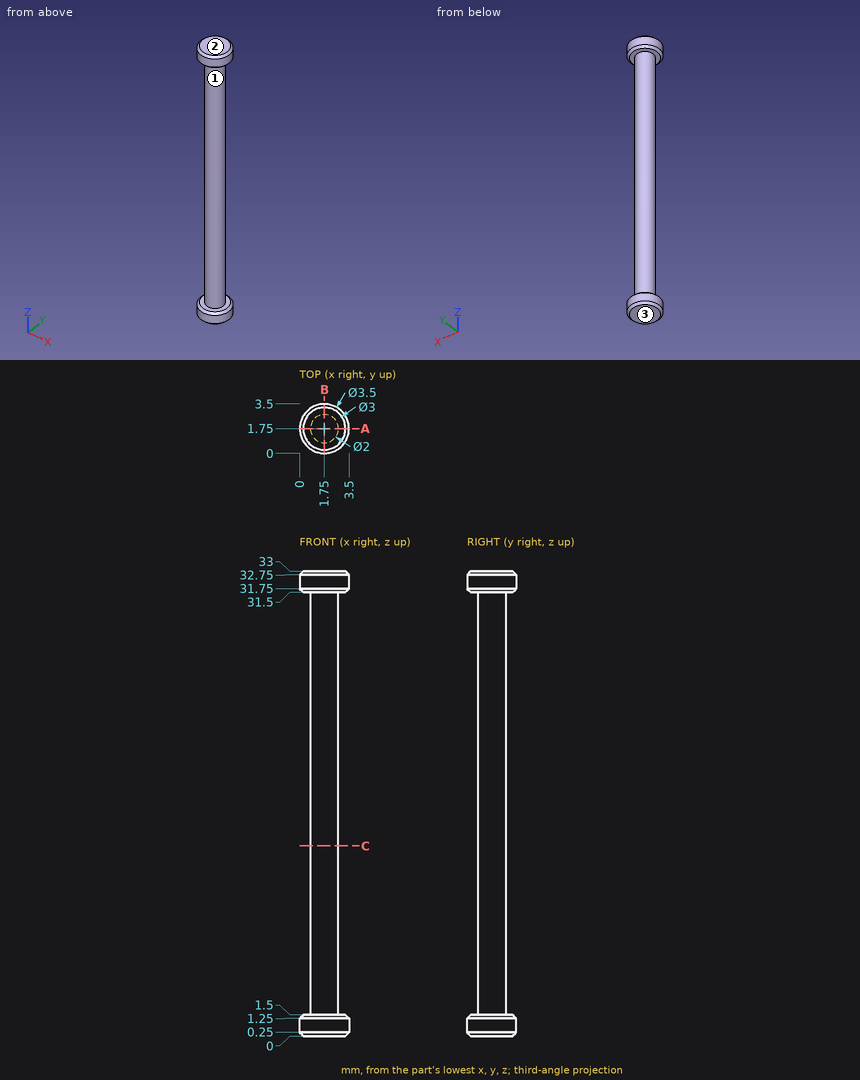
Here's the drawing with two shaded views (mm, measured from the low corner). I have some questions. Round coordinates to 2 decimals unless told otherwise and drop trailing zeros. Loops run counter-clockwise (first coordinate to the right, second up) from the corner with the lowest first, then second, coordinate; pieces in that order, holes last. Notation, with made-up numbers: (17.5, 82.25) - (64.5, 82.25) arc R15 ccw to (64.5, 109.25) - close; hole circle Ø8 at (-31, -21.75). An arc over 180 degrees is marked (long way). Write item = value, one per line.
1) Imagine slicing it at C-C (z = 13.5). Please give me the cut outline in (x, y), and give its area (3 significant figures).
Computed:
outline = circle Ø2 at (1.75, 1.75)
area = 3.14 mm2
2) I'm going to push flat-ended pins straight in: P1, Ø2, axis at y = 2.5, z = 19.5, coming from the -X side; P2, Ø1, axis at y = 2, z = 17, coming from the +X side. Where does each tip first touch, or does it pass through?
Computed:
P1 = 0.75
P2 = 2.75
3) Imagine slicing it at A-A (y = 1.75). Please give me the cut outline in (x, z), and give its area (4 significant figures).
Computed:
outline = (0, 0.25) - (0.25, 0) - (3.25, 0) - (3.5, 0.25) - (3.5, 1.25) - (3.25, 1.5) - (2.75, 1.5) - (2.75, 31.5) - (3.25, 31.5) - (3.5, 31.75) - (3.5, 32.75) - (3.25, 33) - (0.25, 33) - (0, 32.75) - (0, 31.75) - (0.25, 31.5) - (0.75, 31.5) - (0.75, 1.5) - (0.25, 1.5) - (0, 1.25) - close
area = 70.25 mm2
4) I need wall thicknesses on line 1 along Z through (x, y) = (0.6, 1.1); line 2 along X through (y, z) = (1.7, 10.5); line 3 along Y through (x, z) = (1.2, 28.5). Which ranges of each line are inside material? Lowest first, please. Write a range as from..to.
Computed:
line_1 = 0..1.5, 31.5..33
line_2 = 0.75..2.75
line_3 = 0.91..2.59
5) If we mould it in two halves opening along Z, with no side actions, what happens to the marked faces 1, 2 and 3? For each: pulls with the +Z half, pulls with the -Z half, needs draft (parallel to the pull), parting line crosses it, or undercut.
Computed:
face_1 = undercut
face_2 = pulls with the +Z half
face_3 = pulls with the -Z half
